Can you work these out from the drawing? Everything is in mm from the part's minimum corner. Round coordinates to 2 decimals unless told otherwise and drop trailing zeros. Write each loop counter-clockwise with the first axis right and the second up, starting at its lowest first coordinate (ties: lowest second). Pieces come first, ordered by that corner, then holes. Notation, with made-up numbers: (22.25, 7.5) - (48.25, 7.5) arc R25 cw to (48.25, 24.5) - close; hole circle Ø3 at (84.5, -35). An arc over 180 degrees is marked (long way). One line per item, written item: value. Start each with the question number.
Item 1: Imagine slicing it at D-D, the plane z = 12. Please give me the cut outline in (x, y).
Item 2: Thinking about a two-plate mould opening in Z: for the marked faces 1, 2 and 3, which applies, released by +Z, released by -Z, zero draft, split by the parting line, or undercut?
Item 3: Imagine slicing it at B-B, the plane y = 11. Please give me the cut outline in (x, z), then the cut area to 3 significant figures.
Item 4: For P1, Ø18, axis at x = 17.5, y = 29, coming from the +Z side; P2, Ø6, axis at y = 29.5, z = 53, coming from the +X side; P3, Ø4, axis at y = 34.5, z = 13, coming from the +X side; P4, Ø6, axis at x = 25.5, z = 24.5, coming from the -Y side, each with a flat end and sliding along its axis, tell me the tip position at first contact or that it passes through.
Item 5: Imagine slicing it at A-A, the plane x = 30. Please give me the cut outline in (y, z).
Item 6: Imagine slicing it at C-C, the plane x = 10. Please give me the cut outline in (y, z).
Item 7: If I drill on line 1 (Y direction, x = 30, z = 3); line 2 (Z direction, x = 23.5, y = 9.5); line 3 (Y direction, x = 10, z = 3), over which ranges is the centre line in solid material (lowest first)?
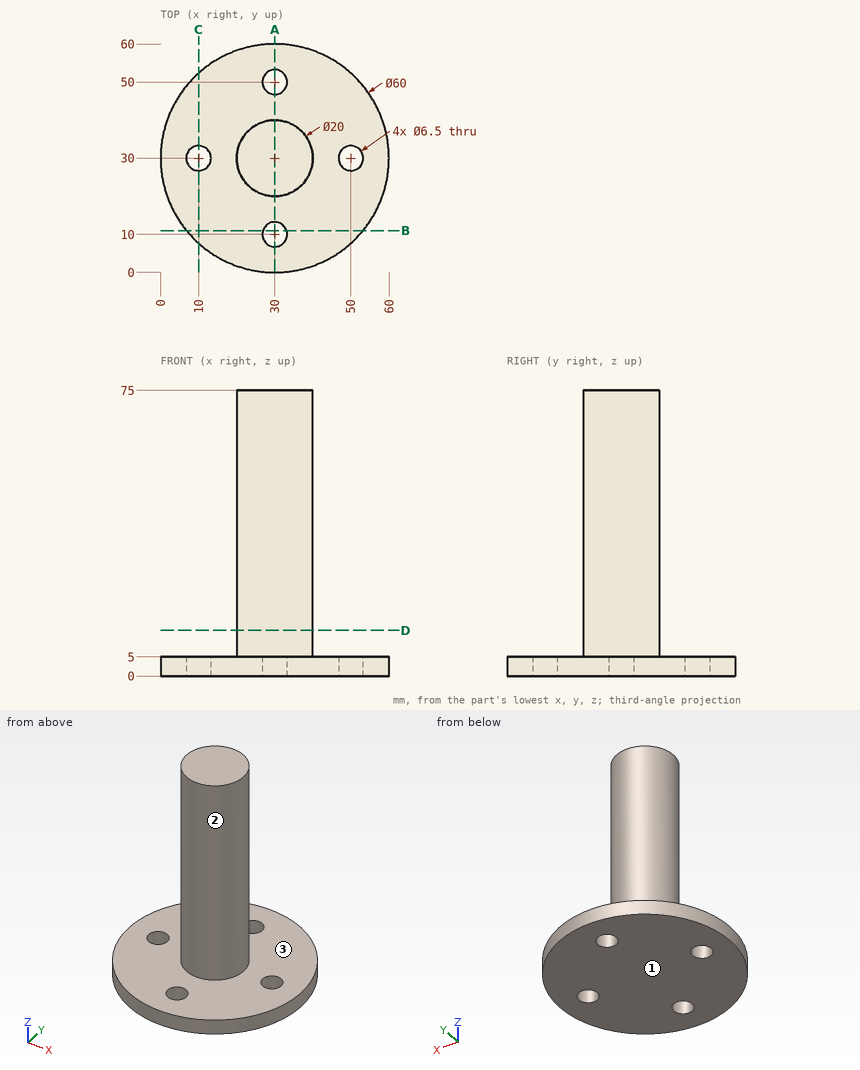
Values follow:
1. outline: circle Ø20 at (30, 30)
2. face 1: released by -Z
2. face 2: zero draft
2. face 3: released by +Z
3. outline: (6.78, 0) - (26.91, 0) - (26.91, 5) - (6.78, 5) - close; (33.09, 0) - (53.22, 0) - (53.22, 5) - (33.09, 5) - close
3. area: 201 mm^2
4. P1: stops at z = 75
4. P2: stops at x = 40
4. P3: stops at x = 39.68
4. P4: stops at y = 20.11
5. outline: (0, 0) - (6.75, 0) - (6.75, 5) - (0, 5) - close; (13.25, 0) - (46.75, 0) - (46.75, 5) - (40, 5) - (40, 75) - (20, 75) - (20, 5) - (13.25, 5) - close; (53.25, 0) - (60, 0) - (60, 5) - (53.25, 5) - close
6. outline: (7.64, 0) - (26.75, 0) - (26.75, 5) - (7.64, 5) - close; (33.25, 0) - (52.36, 0) - (52.36, 5) - (33.25, 5) - close
7. line 1: y = 0 to 6.75, 13.25 to 46.75, 53.25 to 60
7. line 2: z = 0 to 5
7. line 3: y = 7.64 to 26.75, 33.25 to 52.36
